For this review, take the finished solid that the model builds, in its own axes (mm). Coordinates: 2 decimals unless noted, no trailing zeros. Write each loop counter-clockwise with the first axis right and the second up, starting at its lowest first coordinate (ties: lowest second). Pieces come first, ordered by that corner, then holes. Notation, with made-up numbers: (-27, 79.25) -> (-18, 79.25) arc R15 ccw to (-18, 105.25) -> close; hole circle Ø1 at (-2, 58.5). An arc over 180 degrees is marked (long way). Put each result on its own line as item: value. Start each with the question number.
Item 1: Consider section A-A on y = 0. Give the boundary of the cut face in (x, z).
Item 2: Insertion check: P1, Ø2, axis at y = 10, z = 11, coming from the +X side; P2, Ø3, axis at x = 22.5, y = -15.5, coming from the +Z side. Each pin has a flat end and moves straight along its axis. Give the tip position at first contact, or say it passes through.
Item 3: Consider section B-B on x = 25. Give the number of separate pieces and of enclosed holes in the cut face, and give its area (3 significant figures).
Item 4: To check wall thickness, follow L1, parallel to Z at x = 17.2, y = 0; L2, parallel to X at y = 0.5, z = 9.75. State the ranges of each line that lie inside material, in increasing order.
Item 5: Consider section C-C on y = 5. Give the boundary of the cut face in (x, z).
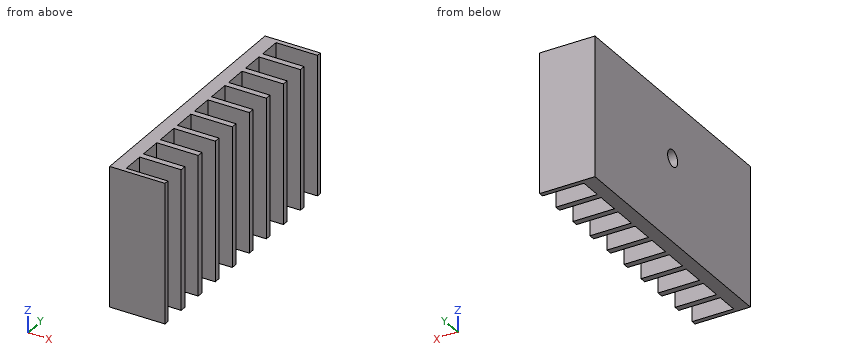
```python
from build123d import *

# Parameters (mm, degrees)
SKETCH002_W     = 10
SKETCH002_H     = 46.5
PAD001_DEPTH    = 25.25
SKETCH003_W     = 10
SKETCH003_H     = 4
POCKET001_DEPTH = 25.25
SKETCH004_R     = 1.5
POCKET002_DEPTH = 5


with BuildPart() as part:
    # Sketch002 → Pad001 (new body)
    with BuildSketch(Plane.XY):
        Rectangle(SKETCH002_W, SKETCH002_H)
    extrude(amount=PAD001_DEPTH)

    # Sketch003 (on Face6 of Pad001) → Pocket001 (cut)
    with BuildSketch(Plane.XY.offset(25.25)):
        with Locations((2.5, 20.4)):
            Rectangle(SKETCH003_W, SKETCH003_H)
        with Locations((2.5, 10.2)):
            Rectangle(SKETCH003_W, SKETCH003_H)
        with Locations((2.5, 15.3)):
            Rectangle(SKETCH003_W, SKETCH003_H)
        with Locations((2.5, 5.1)):
            Rectangle(SKETCH003_W, SKETCH003_H)
        with Locations((2.5, 0)):
            Rectangle(SKETCH003_W, SKETCH003_H)
        with Locations((2.5, -20.4)):
            Rectangle(SKETCH003_W, SKETCH003_H)
        with Locations((2.5, -15.3)):
            Rectangle(SKETCH003_W, SKETCH003_H)
        with Locations((2.5, -10.2)):
            Rectangle(SKETCH003_W, SKETCH003_H)
        with Locations((2.5, -5.1)):
            Rectangle(SKETCH003_W, SKETCH003_H)
    extrude(amount=-POCKET001_DEPTH, mode=Mode.SUBTRACT)

    # Sketch004 (on Face26 of Pocket001) → Pocket002 (cut)
    with BuildSketch(Plane.YZ.offset(-2.5)):
        with Locations((0, 15)):
            Circle(SKETCH004_R)
    extrude(amount=-POCKET002_DEPTH, mode=Mode.SUBTRACT)


with BuildPart() as part_1:
    # Body001 placement: moved
    add(part.part.moved(Location((21.25, 0, 1.65))))


solid = part_1.part
```
Return value:
1. outline: (16.25, 1.65) -> (18.75, 1.65) -> (18.75, 15.15) -> (16.25, 15.15) -> close; (16.25, 18.15) -> (18.75, 18.15) -> (18.75, 26.9) -> (16.25, 26.9) -> close
2. P1: x = 18.75
2. P2: through
3. separate pieces: 10
3. enclosed holes: 0
3. area: 265 mm^2
4. L1: 1.65 to 15.15, 18.15 to 26.9
4. L2: 16.25 to 18.75
5. outline: (16.25, 1.65) -> (18.75, 1.65) -> (18.75, 26.9) -> (16.25, 26.9) -> close
